```python
from build123d import *

# Parameters (mm, degrees)
SKETCH1_R      = 0.635
EXTRUDE1_DEPTH = 3.175
SKETCH2_R      = 1.905
EXTRUDE2_DEPTH = 4.175


with BuildPart() as part:
    # Sketch1 → Extrude1 (new body)
    with BuildSketch(Plane.XY):
        with BuildLine():
            Line((-7.62, 0), (7.62, 0))
            Line((7.62, 0), (7.62, 3.272777676))
            ThreePointArc((7.62, 3.272777676), (8.25562747, 6.041973695), (10.035258768, 8.256783238))
            Line((10.035258768, 8.256783238), (20.079071056, 16.186108729))
            ThreePointArc((20.079071056, 16.186108729), (22.036906124, 23.536555615), (15.53898187, 27.491194408))
            ThreePointArc((15.53898187, 27.491194408), (11.961099032, 26.970268702), (8.451534603, 26.101035293))
            ThreePointArc((8.451534603, 26.101035293), (6.615319821, 25.206255275), (5.1581845, 23.774797045))
            Line((5.1581845, 23.774797045), (-5.161343447, 9.702713481))
            ThreePointArc((-5.161343447, 9.702713481), (-6.989694731, 6.143656664), (-7.62, 2.192394953))
            Line((-7.62, 2.192394953), (-7.62, 0))
        make_face()
        with Locations((-4.7625, 3.175)):
            Circle(SKETCH1_R, mode=Mode.SUBTRACT)
        with Locations(Location((4.7625, 3.175, 0), (0, 0, 180))):  # turned: the seam where the file's is
            Circle(SKETCH1_R, mode=Mode.SUBTRACT)
    extrude(amount=EXTRUDE1_DEPTH)

    # Sketch2 → Extrude2 (cut, through all)
    with BuildSketch(Plane.XY.offset(3.175)):
        with Locations((16.144329824, 21.17011429)):
            Circle(SKETCH2_R)
    extrude(amount=-EXTRUDE2_DEPTH, mode=Mode.SUBTRACT)


solid = part.part
```
Verification items for the finished model (mm, model axes). A direction names the side the tool comes from. Give positions to 0.01 mm unless a question says otherwise; leave off trailing zeros. Order: outer loops, then holes, each group sorted by start corner. A loop starts at its lowest first (then second) coordinate and runs counter-clockwise, first axis right, second up. Notation, with made-up numbers: M 41.5,22 L 89.5,22 A29 ccw 89.5,51 Z; hole C 67.25,75.25 d11. An arc over 180 degrees is marked long. Return JSON: item names as keys, results as strings. Group by question number.
1) Section check D-D on y = 15.5. Record the cut outline in (x, z) (3 decimals), and give its area (3 significant figures).
2) Section check B-B on x = 16.5. Record the cut outline in (y, z) (3 decimals).
3) Go/stop test with flat-tipped pins: pin 1 Ø1 at (x, z) = (18, 1.5) entering from +Y; pin 2 Ø1.5 at (x, z) = (16, 1.5) entering from -Y; pin 3 Ø1 at (y, z) = (6.5, 2.5) entering from +X. Record where each tip stops, or that it passes through.
4) Section check A-A on y = 21.5. Record the cut outline in (x, z) (3 decimals).
5) Section check C-C on z = 0.75. Give the number of separate pieces and of enclosed holes in the cut face, and give its area (3 significant figures).
6) Scan lines: line 1 (X direction, y = 2.25, z = 0.9); line 2 (Y direction, x = 5, z = 2.3); line 3 (X direction, y = 14.5, z = 2.7). Record each from-to range of solid material in increasing order.
7) Access from +Z, -Z, +X, -X, +Y, -Y to the whole of each face (thin tool, end or side, straight path). Record for faces 5 (the face through (-7.62, 1, 2)), 6 (the face through (7.62, 2, 2)).
8) Mould release check, pull along Y, two halves, no side actions. Record for faces 1 (the face through (14.24, 21.25, 1.61)), 2 (the face through (7, 14, 3.175)), 3 (the face through (0.071, 16.837, 1.565)), 4 (the face through (-4.845, 3.805, 1.565)): pulls with the +Y half, pulls with the -Y half, needs draft (parallel to the pull), parting line crosses it, or undercut.
Answer block:
{
 "1": {"outline": "M -0.91,0 L 19.21,0 L 19.21,3.175 L -0.91,3.175 Z", "area": "63.9 mm^2"},
 "2": {"outline": "M 13.361,0 L 19.299,0 L 19.299,3.175 L 13.361,3.175 Z; M 23.042,0 L 27.51,0 L 27.51,3.175 L 23.042,3.175 Z"},
 "3": {"pin 1": "stops at y = 27.37", "pin 2": "stops at y = 12.37", "pin 3": "stops at x = 8.83"},
 "4": {"outline": "M 3.49,0 L 14.268,0 L 14.268,3.175 L 3.49,3.175 Z; M 18.021,0 L 22.486,0 L 22.486,3.175 L 18.021,3.175 Z"},
 "5": {"separate pieces": "1", "enclosed holes": "3", "area": "452 mm^2"},
 "6": {"line 1": "x = -7.62 to 7.62", "line 2": "y = 0 to 2.59, 3.76 to 23.56", "line 3": "x = -1.64 to 17.94"},
 "7": {"face 5": "+Z, -Z, -X, +Y, -Y", "face 6": "+Z, -Z, +X, -Y"},
 "8": {"face 1": "undercut", "face 2": "needs draft", "face 3": "pulls with the +Y half", "face 4": "undercut"}
}
